Geometry: final body of the model. Coordinates: model frame, mm. Face numbers are marked on the shaded views. A direction names the side the tool comes from. Coordinates: 2 decimals unless noted, no trailing zeros. Order: outer loops, then holes, each group sorted by start corner. A loop starts at its lowest first (then second) coordinate and runs counter-clockwise, first axis right, second up. Notation, with made-up numbers: (25.5, -31.75) -> (53.5, -31.75) arc R18 cw to (53.5, -18.75) -> close; hole circle Ø7 at (84, 25.5). An arc over 180 degrees is marked (long way). Answer in a Markdown table with one row per item. Add a question column.
1) Set-up query: the marked faces 4, 5 and 6. Return all of +Z, -Z, +X, -X, +Y, -Y with unobstructed straight access to the full face (end or side cutting, diameter ignored); none if empty.
2) Ray query, line 1 (Y direction, x = 12.5, z = -14.7); line 2 (Z direction, x = 2, y = -2.5); line 3 (Z direction, x = 11.5, y = -100). Return the intervals inside material, ascending. Write a range as from..to.
3) Section query A-A on y = 0. Return the cut outline in (x, z) (3 decimals), then the cut area to 3 significant figures.
4) Section query B-B on x = 5. Return the cut outline in (y, z).
5) Section query C-C on z = 15. Return the cut outline in (x, y) (3 decimals), then the cut area to 3 significant figures.
6) Section query D-D on z = 3.5. Return the cut outline in (x, y) (3 decimals), then the cut area to 3 significant figures.
7) Contact query for flat-ended pins moving along their axis: P1, Ø12, axis at y = -76, z = 4.5, coming from the +X side (3 decimals); P2, Ø2, axis at y = -101, z = -16, coming from the -X side; P3, Ø8, axis at x = 2.5, y = 16, coming from the +Z side. Output: stop coordinate, or through.
8) Pull-direction query (Z, two-part tool) for the marked faces 1, 2 and 3; classes: +Z half, -Z half, draft (parallel to the pull), parting line (faces both ways), or undercut.
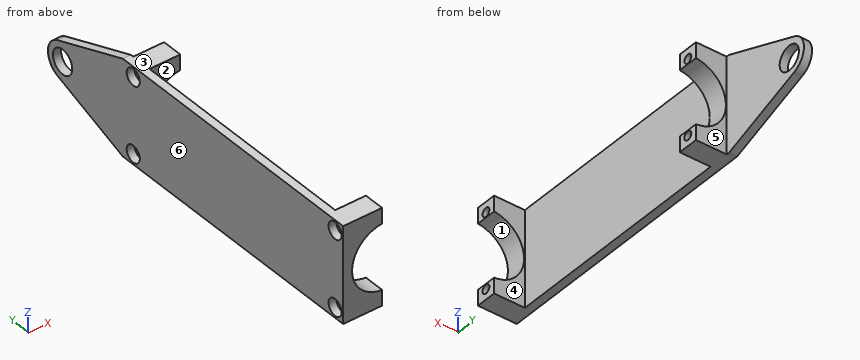
```python
from build123d import *

# Parameters (mm, degrees)
SKETCH1_R                      = 4.7625
BOSS_EXTRUDE1_DEPTH            = 3.175
SKETCH2_W                      = 37.4
SKETCH2_H                      = 8
BOSS_EXTRUDE2_DEPTH            = 12
CUT_EXTRUDE1_DEPTH             = 107.751911575
CUT_EXTRUDE1_DEPTH_BACK        = 107.751911575
SKETCH3_R                      = 12.7
CBORE_FOR_M3_SHCS1_D           = 3.4
CBORE_FOR_M3_SHCS1_CBORE_D     = 6.5
CBORE_FOR_M3_SHCS1_CBORE_DEPTH = 3


with BuildPart() as part:
    # Sketch1 → Boss-Extrude1 (new body)
    with BuildSketch(Plane(origin=(0, 0, 0), x_dir=(0, 0, -1), z_dir=(1, 0, 0))):
        with BuildLine():
            Line((-18.7, -104), (18.7, -104))
            Line((18.7, -104), (18.7, 5.15))
            Line((18.7, 5.15), (6.817247269, 37.503806287))
            ThreePointArc((6.817247269, 37.503806287), (0, 42.2625), (-6.817247269, 37.503806287))
            Line((-6.817247269, 37.503806287), (-18.7, 5.15))
            Line((-18.7, 5.15), (-18.7, -104))
        make_face()
        with Locations((0, 35)):
            Circle(SKETCH1_R, mode=Mode.SUBTRACT)
    extrude(amount=BOSS_EXTRUDE1_DEPTH)

    # Sketch2 → Boss-Extrude2 (add)
    with BuildSketch(Plane(origin=(3.175, 0, 0), x_dir=(0, 0, -1), z_dir=(1, 0, 0))):
        Rectangle(SKETCH2_W, SKETCH2_H)
        with Locations((0, -100)):
            Rectangle(SKETCH2_W, SKETCH2_H)
    extrude(amount=BOSS_EXTRUDE2_DEPTH)

    # Sketch3 → Cut-Extrude1 (cut, two sides: drawn at the far end of the back side and taken through both)
    with BuildSketch(Plane(origin=(0, 0, 0), x_dir=(1, 0, 0), z_dir=(0, 1, 0)).offset(-CUT_EXTRUDE1_DEPTH_BACK)):
        with Locations((16.175, 0)):
            Circle(SKETCH3_R)
    extrude(amount=CUT_EXTRUDE1_DEPTH + CUT_EXTRUDE1_DEPTH_BACK, mode=Mode.SUBTRACT)

    # CBORE for M3 SHCS1 (through all)
    with Locations(Plane.ZY):
        with Locations((-14.7, 0), (14.7, 0), (14.7, -100), (-14.7, -100)):
            CounterBoreHole(CBORE_FOR_M3_SHCS1_D / 2, CBORE_FOR_M3_SHCS1_CBORE_D / 2, CBORE_FOR_M3_SHCS1_CBORE_DEPTH)


solid = part.part
```
Result:
| question | item | result |
|---|---|---|
| 1 | face 4 | +Z, -Z, +X |
| 1 | face 5 | +Z, -Z, +X, +Y |
| 1 | face 6 | +Z, -Z, -X, +Y, -Y |
| 2 | line 1 | -104..-101.7, -98.3..-96, -4..-1.7, 1.7..4 |
| 2 | line 2 | -18.7..-16.78, -12.62..12.62, 16.78..18.7 |
| 2 | line 3 | -18.7..-16.4, -13..-11.81, 11.81..13, 16.4..18.7 |
| 3 | outline | (0, -18.7) -> (15.175, -18.7) -> (15.175, -16.4) -> (3, -16.4) -> (3, -17.95) -> (0, -17.95) -> close; (0, -11.45) -> (3, -11.45) -> (3, -13) -> (15.175, -13) -> (15.175, -12.661) arc R12.7 cw to (15.175, 12.661) -> (15.175, 13) -> (3, 13) -> (3, 11.45) -> (0, 11.45) -> close; (0, 17.95) -> (3, 17.95) -> (3, 16.4) -> (15.175, 16.4) -> (15.175, 18.7) -> (0, 18.7) -> close |
| 3 | area | 218 mm2 |
| 4 | outline | (-104, -18.7) -> (-96, -18.7) -> (-96, -6.03) -> (-104, -6.03) -> close; (-104, 6.03) -> (-96, 6.03) -> (-96, 18.7) -> (-104, 18.7) -> close; (-4, -18.7) -> (4, -18.7) -> (4, -6.03) -> (-4, -6.03) -> close; (-4, 6.03) -> (4, 6.03) -> (4, 18.7) -> (-4, 18.7) -> close; hole circle Ø3.4 at (-100, -14.7); hole circle Ø3.4 at (-100, 14.7); hole circle Ø3.4 at (0, -14.7); hole circle Ø3.4 at (0, 14.7) |
| 5 | outline | (0, -104) -> (15.175, -104) -> (15.175, -101.673) -> (3, -101.673) -> (3, -103.236) -> (0, -103.236) -> close; (0, -96.764) -> (3, -96.764) -> (3, -98.327) -> (15.175, -98.327) -> (15.175, -96) -> (3.175, -96) -> (3.175, -4) -> (15.175, -4) -> (15.175, -1.673) -> (3, -1.673) -> (3, -3.236) -> (0, -3.236) -> close; (0, 3.236) -> (3, 3.236) -> (3, 1.673) -> (15.175, 1.673) -> (15.175, 4) -> (3.175, 4) -> (3.175, 15.224) -> (0, 15.224) -> close |
| 5 | area | 450 mm2 |
| 6 | outline | (0, -104) -> (3.967, -104) -> (3.967, -96) -> (3.175, -96) -> (3.175, -4) -> (3.967, -4) -> (3.967, 4) -> (3.175, 4) -> (3.175, 31.77) -> (0, 31.77) -> close; (0, 38.23) -> (3.175, 38.23) -> (3.175, 41.363) -> (0, 41.363) -> close |
| 6 | area | 454 mm2 |
| 7 | P1 | x = 3.175 |
| 7 | P2 | x = 3 |
| 7 | P3 | z = 16.18 |
| 8 | face 1 | undercut |
| 8 | face 2 | draft |
| 8 | face 3 | +Z half |
